The model under review builds one solid part; all positions refer to its coordinate system, in mm. A direction names the side the tool comes from. Give positions to 0.01 mm unless a question says otherwise; leave off trailing zeros. Loops run counter-clockwise (first coordinate to the right, second up) from the corner with the lowest first, then second, coordinate; pieces in that order, holes last. Notation, with made-up numbers: M -31,60.5 L 22,60.5 A20 cw 22,91.5 Z; hole C 2,85.25 d7. An arc over 180 degrees is marked long. One line per item, written item: value. Start each with the question number.
Q1. To check wall thickness, follow line 1 along Z through (x, y) = (1.95, 0); line 2 along Y through (x, z) = (4, 32); line 3 along Z through (x, y) = (4.3, 8). State the ranges of each line that lie inside material, in increasing order. Write a range as from..to.
Q2. Mouldability with a two-part tool opening along Y and no side actions: class faces 1 (the face through (24, 0, 0)), 2 (the face through (3.084, -0.521, 35.966)), 3 (the face through (13, 16, 12)), 4 (the face through (4.45, -8.46, 35.47)) as released by +Y, released by -Y, zero draft, split by the parting line, or undercut.
Q3. We need section D-D on x = 5. Write out the cut boundary in (y, z).
Q4. We need section C-C on z = 40. Write out the cut boundary in (x, y).
Q5. For faces 5 (the face through (39, 0, 6)), 6 (the face through (2.8, 10, 30)), 7 (the face through (13, -16, 12)), list the 3-axis set-ups (+Z, -Z, +X, -X, +Y, -Y) from which the entire face can be reached by the end or side of a thin tool; tool diameter is ignored.
Q6. For pin 1 (6.5 mm diameter, centred on y = 0, z = 24, fed in from +X); pin 2 (9 mm diameter, centred on y = 0, z = 32, fed in from +X); pin 3 (3.5 mm diameter, centred on y = 1.5, z = 38.5, fed in from +X), all flat-tipped, find the tip position at first contact; note any pin that passes through.
Q7. We need section B-B on y = 8. Write out the cut boundary in (x, z).
Q8. We need section A-A on z = 32. Write out the cut boundary in (x, y).
```python
from build123d import *

# Parameters (mm, degrees)
F5_DEPTH      = 16
F7_R          = 24
F6_R          = 2
F6_R_2        = 4
F8_DEPTH      = 6.001
F8_DEPTH_BACK = 42.001
F6_R_3        = 3.5
F9_DEPTH      = 3.2
F9_DEPTH_BACK = 42.001


with BuildPart() as f5:
    # F4 (on Front) → F5 (new body, symmetric)
    with BuildSketch(Plane.XZ):
        Polygon((6, 48), (0, 48), (0, 0), (48, 0), (48, 6), (6, 6), align=None)
    extrude(amount=F5_DEPTH, both=True)

    # F7
    f7_edges = [f5.edges().sort_by_distance(p)[0] for p in [
        (6, 0, 6),
    ]]
    fillet(f7_edges, radius=F7_R)

    # F6 (on face) → F8 (cut, two sides)
    with BuildSketch(Plane.YZ.offset(6)) as f8_sk:
        with Locations((-8, 32)):
            Circle(F6_R)
        with Locations((0, 40)):
            Circle(F6_R)
        with Locations((8, 32)):
            Circle(F6_R)
        with Locations((0, 32)):
            Circle(F6_R_2)
        with Locations((0, 24)):
            Circle(F6_R)
    extrude(amount=-F8_DEPTH, mode=Mode.SUBTRACT)
    extrude(f8_sk.sketch, amount=F8_DEPTH_BACK, mode=Mode.SUBTRACT)

    # F6 (on face) → F9 (cut, two sides)
    with BuildSketch(Plane.YZ.offset(6)) as f9_sk:
        with Locations((-8, 32)):
            Circle(F6_R_3)
        with Locations((-8, 32)):
            Circle(F6_R, mode=Mode.SUBTRACT)
        with Locations((0, 40)):
            Circle(F6_R_3)
        with Locations((0, 40)):
            Circle(F6_R, mode=Mode.SUBTRACT)
        with Locations((8, 32)):
            Circle(F6_R_3)
        with Locations((8, 32)):
            Circle(F6_R, mode=Mode.SUBTRACT)
        with Locations((0, 24)):
            Circle(F6_R_3)
        with Locations((0, 24)):
            Circle(F6_R, mode=Mode.SUBTRACT)
    extrude(amount=-F9_DEPTH, mode=Mode.SUBTRACT)
    extrude(f9_sk.sketch, amount=F9_DEPTH_BACK, mode=Mode.SUBTRACT)


solid = f5.part
```
Solved:
1. line 1: 0..22, 26..28, 36..38, 42..48
1. line 2: -16..-11.5, -4.5..-4, 4..4.5, 11.5..16
1. line 3: 0..28.5, 35.5..48
2. face 1: zero draft
2. face 2: undercut
2. face 3: released by +Y
2. face 4: undercut
3. outline: M -16,0 L 16,0 L 16,48 L -16,48 Z; hole C -8,32 d7; hole C 0,32 d8; hole C 0,24 d7; hole C 0,40 d7; hole C 8,32 d7
4. outline: M 0,-16 L 6,-16 L 6,-3.5 L 2.8,-3.5 L 2.8,-2 L 0,-2 Z; M 0,2 L 2.8,2 L 2.8,3.5 L 6,3.5 L 6,16 L 0,16 Z
5. face 5: +Z, +X, +Y, -Y
5. face 6: +X
5. face 7: +Z, -Z, +X, -X, -Y
6. pin 1: x = 2.8
6. pin 2: x = 6.13
6. pin 3: x = 6
7. outline: M 0,0 L 48,0 L 48,6 L 30,6 A24 cw 6.05,28.5 L 2.8,28.5 L 2.8,30 L 0,30 Z; M 0,34 L 2.8,34 L 2.8,35.5 L 6,35.5 L 6,48 L 0,48 Z
8. outline: M 0,-16 L 6,-16 L 6,-11.5 L 2.8,-11.5 L 2.8,-10 L 0,-10 Z; M 0,-6 L 2.8,-6 L 2.8,-4.5 L 6,-4.5 L 6,-4 L 0,-4 Z; M 0,4 L 6,4 L 6,4.5 L 2.8,4.5 L 2.8,6 L 0,6 Z; M 0,10 L 2.8,10 L 2.8,11.5 L 6,11.5 L 6,16 L 0,16 Z
